from build123d import *

# Parameters (mm, degrees)
ESQUISSE1_R        = 18.75
ESQUISSE1_R_2      = 15.5
BOSS_EXTRU_1_DEPTH = 12
CONG_1_R           = 0.5


with BuildPart() as part:
    # Esquisse1 → Boss.-Extru.1 (new body)
    with BuildSketch(Plane(origin=(0, 0, 0), x_dir=(1, 0, 0), z_dir=(0, 1, 0))):
        with Locations(Location((0, 0, 0), (0, 0, 270))):  # turned: the seam where the file's is
            Circle(ESQUISSE1_R)
        with Locations(Location((0, 0, 0), (0, 0, 270))):  # turned: the seam where the file's is
            Circle(ESQUISSE1_R_2, mode=Mode.SUBTRACT)
    extrude(amount=BOSS_EXTRU_1_DEPTH)

    # Congé1
    cong_1_edges = [part.edges().sort_by_distance(p)[0] for p in [
        (0, 0, -18.75),
        (0, 12, -18.75),
        (0, 0, -15.5),
        (0, 12, -15.5),
    ]]
    fillet(cong_1_edges, radius=CONG_1_R)


solid = part.part
Source: CAD feature listing. Evaluate the final solid. Frame: model axes, mm. Round coordinates to 2 decimals unless told otherwise and drop trailing zeros. Order: outer loops, then holes, each group sorted by start corner. A loop starts at its lowest first (then second) coordinate and runs counter-clockwise, first axis right, second up. Notation, with made-up numbers: (82.5, -2.5) - (134.5, -2.5) arc R32 ccw to (134.5, 27.5) - close; hole circle Ø11 at (59.25, 0.5). An arc over 180 degrees is marked (long way). Use a Markdown table: item, result. Add a question column.
1. Line query: probe 1 along X at (y, z) = (10.5, 0.5); probe 2 along Z at (x, y) = (12, 4.5); probe 3 along Z at (x, y) = (2, 4.25). Output: solid intervals per line, ascending.
2. Mould query, pull axis Z, two halves, no side actions, for faces 1 (the cylindrical face through (15.368, 5.923, -2.018)), 2 (the cylindrical face through (-11.41, 5.92, -14.88)), 3 (the flat face through (-16.1, 12, 1.3)). Classes: +Z half, -Z half, draft (parallel to the pull), parting line (faces both ways), or undercut.
3. Section query A-A (x = 0). Return the cut outline in (y, z).
4. First-contact query: pin 1 (6 mm diameter, centred on y = 8, z = 14.5, fed in from -X); pin 2 (3 mm diameter, centred on y = 3.5, z = 8.5, fed in from +X); pin 3 (2 mm diameter, centred on x = 14.5, z = 2.5, fed in from -Y); pin 4 (4 mm diameter, centred on x = -2, y = 5.5, fed in from +Z). Flat tips, straight axial feed; report the tip coordinate or a pass-through.
5. Section query B-B (z = 0). Return the cut outline in (x, y), then the cut area to 3 significant figures.
6. Section query C-C (y = 3.25). Return the cut outline in (x, z), then the cut area to 3 significant figures.
Derived:
| question | item | result |
|---|---|---|
| 1 | probe 1 | -18.74 to -15.49, 15.49 to 18.74 |
| 1 | probe 2 | -14.41 to -9.81, 9.81 to 14.41 |
| 1 | probe 3 | -18.64 to -15.37, 15.37 to 18.64 |
| 2 | face 1 | undercut |
| 2 | face 2 | parting line |
| 2 | face 3 | draft |
| 3 | outline | (0, -18.25) arc R0.5 ccw to (0.5, -18.75) - (11.5, -18.75) arc R0.5 ccw to (12, -18.25) - (12, -16) arc R0.5 ccw to (11.5, -15.5) - (0.5, -15.5) arc R0.5 ccw to (0, -16) - close; (0, 16) arc R0.5 ccw to (0.5, 15.5) - (11.5, 15.5) arc R0.5 ccw to (12, 16) - (12, 18.25) arc R0.5 ccw to (11.5, 18.75) - (0.5, 18.75) arc R0.5 ccw to (0, 18.25) - close |
| 4 | pin 1 | x = -14.81 |
| 4 | pin 2 | x = 17.39 |
| 4 | pin 3 | y = 0.09 |
| 4 | pin 4 | z = 18.75 |
| 5 | outline | (-18.75, 0.5) arc R0.5 ccw to (-18.25, 0) - (-16, 0) arc R0.5 ccw to (-15.5, 0.5) - (-15.5, 11.5) arc R0.5 ccw to (-16, 12) - (-18.25, 12) arc R0.5 ccw to (-18.75, 11.5) - close; (15.5, 0.5) arc R0.5 ccw to (16, 0) - (18.25, 0) arc R0.5 ccw to (18.75, 0.5) - (18.75, 11.5) arc R0.5 ccw to (18.25, 12) - (16, 12) arc R0.5 ccw to (15.5, 11.5) - close |
| 5 | area | 77.6 mm2 |
| 6 | outline | circle Ø37.5 at (0, 0); hole circle Ø31 at (0, 0) |
| 6 | area | 350 mm2 |
